Source: CAD feature listing. Evaluate the final solid. Frame: model axes, mm. A direction names the side the tool comes from. Give positions to 0.01 mm unless a question says otherwise; leave off trailing zeros. Write each loop counter-clockwise with the first axis right and the second up, starting at its lowest first coordinate (ties: lowest second). Pieces come first, ordered by that corner, then holes. Notation, with made-up numbers: (67, 2) -> (72, 2) arc R14 cw to (72, 26) -> close; hole circle Ø4 at (-1.5, 67). An arc over 180 degrees is marked (long way). Use a Markdown table: item, result. Add a question column.
```python
from build123d import *

# Parameters (mm, degrees)
SKETCH1_W           = 53.5
SKETCH1_H           = 38.5
BOSS_EXTRUDE1_DEPTH = 2
SKETCH2_W           = 12
SKETCH2_H           = 9.5
BOSS_EXTRUDE2_DEPTH = 3
CUT_EXTRUDE1_DEPTH  = 2


with BuildPart() as part:
    # Sketch1 → Boss-Extrude1 (new body)
    with BuildSketch(Plane(origin=(0, 0, 0), x_dir=(1, 0, 0), z_dir=(0, 1, 0))):
        Rectangle(SKETCH1_W, SKETCH1_H)
    extrude(amount=-BOSS_EXTRUDE1_DEPTH)

    # Sketch2 → Boss-Extrude2 (add)
    # profile 1 of 2: a face of its own
    with BuildSketch(Plane(origin=(0, 0, 0), x_dir=(1, 0, 0), z_dir=(0, 1, 0))):
        with Locations((-32.75, 9.5)):
            Rectangle(SKETCH2_W, SKETCH2_H)
        Polygon((-33, 6.440043573), (-30.35, 7.970021787), (-30.35, 11.029978213), (-33, 12.559956427), (-35.65, 11.029978213), (-35.65, 7.970021787), align=None, mode=Mode.SUBTRACT)
    # profile 2 of 2: a face of its own
    with BuildSketch(Plane(origin=(0, 0, 0), x_dir=(1, 0, 0), z_dir=(0, 1, 0))):
        with Locations((32.75, 9.5)):
            Rectangle(SKETCH2_W, SKETCH2_H)
        Polygon((35.65, 7.970021787), (33, 6.440043573), (30.35, 7.970021787), (30.35, 11.029978213), (33, 12.559956427), (35.65, 11.029978213), align=None, mode=Mode.SUBTRACT)
    extrude(amount=-BOSS_EXTRUDE2_DEPTH)

    # Sketch3 → Cut-Extrude1 (cut)
    with BuildSketch(Plane(origin=(0, 0, 0), x_dir=(1, 0, 0), z_dir=(0, 1, 0))):
        with BuildLine():
            Line((-26.75, 4.75), (-26.75, -10.25))
            ThreePointArc((-26.75, -10.25), (-19.25, -2.75), (-26.75, 4.75))
        make_face()
        with BuildLine():
            Line((26.75, 4.75), (26.75, -10.25))
            ThreePointArc((26.75, -10.25), (19.25, -2.75), (26.75, 4.75))
        make_face()
    extrude(amount=-CUT_EXTRUDE1_DEPTH, mode=Mode.SUBTRACT)


solid = part.part
```
(1) Cut plane C-C on x = -32. Return the cut outline in (y, z).
(2) Cut plane B-B on z = 12.5. Return the cut outline in (x, y).
(3) Cut plane D-D on x = 3. Return the cut outline in (y, z), then the cut area to 3 significant figures.
(4) Material intervals for L1, parallel to X at y = -0.45, z = -11; L2, parallel to X at y = -2.15, z = -12.5; L3, parallel to X at y = -1.8, z = -7, sorted ascending.
(5) Cut plane A-A on x = 25. Return the cut outline in (y, z), then the cut area to 3 significant figures.
(6) First-contact query: pin 1 Ø0.9 at (x, y) = (31, -1.5) entering from +Z; pin 2 Ø12 at (x, z) = (-23, 3) entering from -Y; pin 3 Ø8 at (x, z) = (29, 5) entering from +Y; pin 4 Ø1.6 at (y, z) = (-1.5, 13.5) entering from -X. Flat tips, straight axial feed; report the tip coordinate or a pass-through.
(7) Access query for faces 5 (the flat face through (-34.306, -1.479, -11.806)), 6 (the flat face through (26.75, -1, -17)), 7 (the cylindrical face through (19.25, -0.99, 2.91)), 8 (the flat face through (-26.75, -1, -17)), 9 (the flat face through (0, -2, 0)). Directions: +Z, -Z, +X, -X, +Y, -Y. A direction counts if a zero-diameter tool reaches every point of the face in a straight line with its end or side. Return the directions, or none.
(8) Mould query, pull axis Z, two halves, no side actions, for faces 1 (the flat face through (31.656, -1.479, -11.784)), 2 (the flat face through (33, -1, -4.75)), 3 (the flat face through (-33, -1, -14.25)), 4 (the flat face through (31, -3, -12)). Classes: +Z half, -Z half, draft (parallel to the pull), parting line (faces both ways), or undercut.
Output:
| question | item | result |
|---|---|---|
| 1 | outline | (-3, -14.25) -> (0, -14.25) -> (0, -11.98) -> (-3, -11.98) -> close; (-3, -7.02) -> (0, -7.02) -> (0, -4.75) -> (-3, -4.75) -> close |
| 2 | outline | (-26.75, -2) -> (26.75, -2) -> (26.75, 0) -> (-26.75, 0) -> close |
| 3 | outline | (-2, -19.25) -> (0, -19.25) -> (0, 19.25) -> (-2, 19.25) -> close |
| 3 | area | 77.0 mm^2 |
| 4 | L1 | -38.75 to -35.65, -30.35 to 30.35, 35.65 to 38.75 |
| 4 | L2 | -38.75 to -33.1, -32.9 to -26.75, 26.75 to 32.9, 33.1 to 38.75 |
| 4 | L3 | -38.75 to -33.97, -32.03 to 32.03, 33.97 to 38.75 |
| 5 | outline | (-2, -19.25) -> (0, -19.25) -> (0, -4.54) -> (-2, -4.54) -> close; (-2, 10.04) -> (0, 10.04) -> (0, 19.25) -> (-2, 19.25) -> close |
| 5 | area | 47.8 mm^2 |
| 6 | pin 1 | z = -4.75 |
| 6 | pin 2 | y = -2 |
| 6 | pin 3 | through |
| 6 | pin 4 | x = -26.75 |
| 7 | face 5 | +Y, -Y |
| 7 | face 6 | -Z, +X, +Y, -Y |
| 7 | face 7 | +X, +Y, -Y |
| 7 | face 8 | -Z, -X, +Y, -Y |
| 7 | face 9 | +Z, -Z, -Y |
| 8 | face 1 | undercut |
| 8 | face 2 | +Z half |
| 8 | face 3 | -Z half |
| 8 | face 4 | draft |
